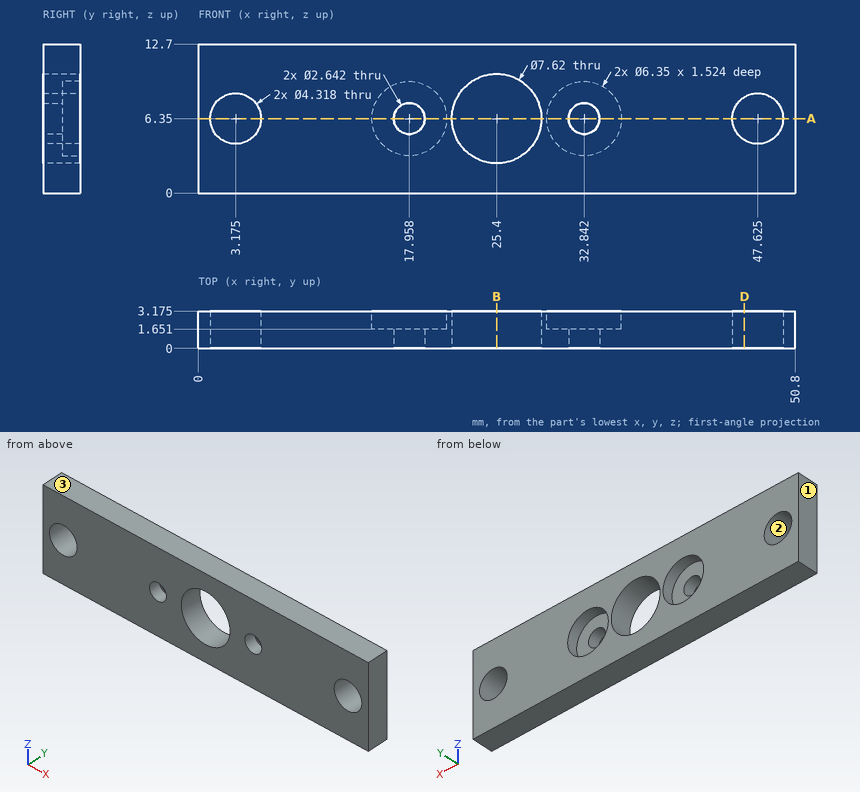
Source: three-view drawing plus pictorial views. Frame: mm from the lowest corner of the part. Give positions to 0.01 mm unless a question says otherwise; leave off trailing zeros. Order: outer loops, then holes, each group sorted by start corner. A loop starts at its lowest first (then second) coordinate and runs counter-clockwise, first axis right, second up. Notation, with made-up numbers: (-10, 22.5) - (5, 22.5) arc R26 cw to (5, 46.5) - close; hole circle Ø7 at (-26.75, 44). An arc over 180 degrees is marked (long way). Answer as a JSON object with one key per item and string values. Group by question number.
Q1. Cut plane D-D, the plane x = 46.5. Output: boundary loops of the cut face in (y, z) (1 decimal).
Q2. First-contact query: pin 1 Ø2.5 at (x, z) = (3.175, 6.35) entering from -Y; pin 2 Ø4 at (x, z) = (17.96, 6.35) entering from +Y. Flat tips, straight axial feed; report the tip coordinate or a pass-through.
Q3. Line query: probe 1 along X at (y, z) = (0.9, 6.35); probe 2 along X at (y, z) = (2.4, 6.35); probe 3 along Z at (x, y) = (27.5, 2.5). Output: solid intervals per line, ascending.
Q4. Cut plane B-B, the plane x = 25.4. Output: boundary loops of the cut face in (y, z) (1 decimal).
Q5. Mould query, pull axis X, two halves, no side actions, for the marked faces 1, 2 and 3. Classes: pulls with the +X half, pulls with the -X half, needs draft (parallel to the pull), parting line crosses it, or undercut.
Q6. Cut plane A-A, the plane z = 6.35. Count the separate pieces of the cut face and the enclosed holes in it.
Results:
{
 "1": {"outline": "(0, 0) - (3.2, 0) - (3.2, 4.5) - (0, 4.5) - close; (0, 8.2) - (3.2, 8.2) - (3.2, 12.7) - (0, 12.7) - close"},
 "2": {"pin 1": "through", "pin 2": "y = 1.65"},
 "3": {"probe 1": "0 to 1.02, 5.33 to 16.64, 19.28 to 21.59, 29.21 to 31.52, 34.16 to 45.47, 49.78 to 50.8", "probe 2": "0 to 1.02, 5.33 to 14.78, 21.13 to 21.59, 29.21 to 29.67, 36.02 to 45.47, 49.78 to 50.8", "probe 3": "0 to 3.17, 9.53 to 12.7"},
 "4": {"outline": "(0, 0) - (3.2, 0) - (3.2, 2.5) - (0, 2.5) - close; (0, 10.2) - (3.2, 10.2) - (3.2, 12.7) - (0, 12.7) - close"},
 "5": {"face 1": "pulls with the -X half", "face 2": "undercut", "face 3": "needs draft"},
 "6": {"separate pieces": "6", "enclosed holes": "0"}
}
